Could you check a few things on this model? Use its own coordinates, in mm. Face numbers are marked on the shaded views. A direction names the side the tool comes from. Give positions to 0.01 mm unless a question says otherwise; leave off trailing zeros. Order: outer loops, then holes, each group sorted by start corner. A loop starts at its lowest first (then second) coordinate and runs counter-clockwise, first axis right, second up. Notation, with made-up numbers: (31.25, 84.5) -> (45.25, 84.5) arc R15 ccw to (45.25, 104.5) -> close; hole circle Ø10 at (-39, 30.25). An arc over 180 degrees is marked (long way). One line per item, written item: value.
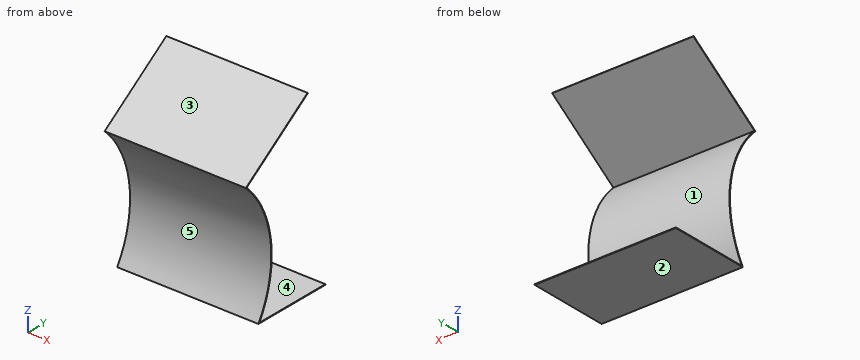
```python
from build123d import *

# Parameters (mm, degrees)
F1_DEPTH = 35.56
F2_SCALE = 10


with BuildPart() as f1:
    # F0 (on Right) → F1 (new body, symmetric)
    with BuildSketch(Plane.YZ):
        with BuildLine():
            Line((-15.24, 0), (25.4, 0))
            Line((25.4, 0), (25.4, 0.3048))
            Line((25.4, 0.3048), (-14.6917010188, 0.3048))
            ThreePointArc((-14.6917010188, 0.3048), (-7.5112329288, 33.2260010127), (-22.3841798034, 63.4610807938))
            Line((-22.3841798034, 63.4610807938), (14.7664575627, 89.4742371269))
            Line((14.7664575627, 89.4742371269), (14.5916314649, 89.72391467))
            Line((14.5916314649, 89.72391467), (-22.86, 63.5))
            ThreePointArc((-22.86, 63.5), (-7.8029756135, 33.0996429264), (-15.24, 0))
        make_face()
    extrude(amount=F1_DEPTH, both=True)


with BuildPart() as f1_1:
    # F2: moved
    add(f1.part.scale(F2_SCALE))


solid = f1_1.part
```
1) For P1, Ø1.5, axis at x = -16.5, z = 610.5, coming from the +Y side; P2, Ø5, axis at x = -246, y = -161, coming from the -Z side; P3, Ø1.5, axis at x = 255.5, z = 440, coming from the -Y side, each with a flat end and sliding along its axis, tell me the tip position at first contact or that it passes through.
Answer below:
P1: stops at y = -200.23
P2: stops at z = 550.41
P3: stops at y = -103.8
2) If I drill on line 1 along Z through (x, y) = (-206.5, -142); line 2 along Z through (x, y) = (-176.5, -48); line 3 along Z through (x, y) = (-181, 200), over which ranges is the centre line in solid material (lowest first)?
Answer below:
line 1: z = 0 to 3.05, 11.23 to 17.29, 523.65 to 529.72, 691.92 to 695.64
line 2: z = 0 to 3.05, 757.74 to 761.46
line 3: z = 0 to 3.05
3) Suppose I cut it at B-B, the plane y = -104.5. Write out the boundary of the cut face in (x, z).
Answer below:
outline: (-355.6, 0) -> (355.6, 0) -> (355.6, 3.05) -> (-355.6, 3.05) -> close; (-355.6, 89.44) -> (355.6, 89.44) -> (355.6, 98.24) -> (-355.6, 98.24) -> close; (-355.6, 442.71) -> (355.6, 442.71) -> (355.6, 451.5) -> (-355.6, 451.5) -> close; (-355.6, 718.17) -> (355.6, 718.17) -> (355.6, 721.9) -> (-355.6, 721.9) -> close
4) For the marked faces 4 and 5, which set-ups out of +Z, -Z, +X, -X, +Y, -Y let a thin tool reach every point of the face, with its end or its side?
Answer below:
face 4: +X, -X, +Y
face 5: +X, -X, -Y
5) We'd pull the mould along Z, two halves only. Please class the marked faces 1, 2 and 3: +Z half, -Z half, draft (parallel to the pull), parting line (faces both ways), or undercut.
Answer below:
face 1: undercut
face 2: -Z half
face 3: +Z half
6) Suppose I cut it at C-C, the plane y = -33. Write out the boundary of the cut face in (x, z).
Answer below:
outline: (-355.6, 0) -> (355.6, 0) -> (355.6, 3.05) -> (-355.6, 3.05) -> close; (-355.6, 768.24) -> (355.6, 768.24) -> (355.6, 771.96) -> (-355.6, 771.96) -> close
7) Suppose I cut it at A-A, the plane x = -141.5. Write out the boundary of the cut face in (y, z), then the cut area to 3 significant figures.
Answer below:
outline: (-228.6, 635) arc R508 cw to (-152.4, 0) -> (254, 0) -> (254, 3.05) -> (-146.92, 3.05) arc R511.05 ccw to (-223.84, 634.61) -> (147.66, 894.74) -> (145.92, 897.24) -> close
area: 4,720 mm2
